Design review of the part built by this model. Coordinates are the model's own, in mm. A direction names the side the tool comes from. Give positions to 0.01 mm unless a question says otherwise; leave off trailing zeros. Order: outer loops, then holes, each group sorted by start corner. A loop starts at its lowest first (then second) coordinate and runs counter-clockwise, first axis right, second up. Notation, with made-up numbers: M -29.75,11 L -9.75,11 A18 ccw -9.75,36 Z; hole C -37,74 d1. An arc over 180 degrees is marked long. Answer as a JSON object with one key per item and string values.
from build123d import *

# Parameters (mm, degrees)
SKETCH_2_W          = 50
SKETCH_2_H          = 60
EXTRUDE_1_DEPTH     = 5
SKETCH_3_W          = 5
SKETCH_3_H          = 60
EXTRUDE_2_DEPTH     = 80
EXTRUDE_3_DEPTH     = 10
EXTRUDE_4_DEPTH     = 10
EXTRUDE_5_DEPTH     = 5
SKETCH_7_R          = 1.55
CUT_EXTRUDE_1_DEPTH = 112.803398875


with BuildPart() as part:
    # 草图2 → 凸台-拉伸1 (new body)
    with BuildSketch(Plane(origin=(0, 0, 0), x_dir=(1, 0, 0), z_dir=(0, 1, 0))):
        with Locations((25, 30)):
            Rectangle(SKETCH_2_W, SKETCH_2_H)
    extrude(amount=EXTRUDE_1_DEPTH)

    # 草图3 → 凸台-拉伸2 (add)
    with BuildSketch(Plane(origin=(0, 5, 0), x_dir=(1, 0, 0), z_dir=(0, 1, 0))):
        with Locations((47.5, 30)):
            Rectangle(SKETCH_3_W, SKETCH_3_H)
    extrude(amount=EXTRUDE_2_DEPTH)

    # 草图4 → 凸台-拉伸3 (add)
    with BuildSketch(Plane.XY):
        Polygon((39, 5), (45, 25), (45, 5), align=None)
    extrude(amount=-EXTRUDE_3_DEPTH)

    # 草图5 → 凸台-拉伸4 (add)
    with BuildSketch(Plane(origin=(0, 0, -60), x_dir=(-1, 0, 0), z_dir=(0, 0, -1))):
        Polygon((-39, 5), (-45, 25), (-45, 5), align=None)
    extrude(amount=-EXTRUDE_4_DEPTH)

    # 草图6 → 凸台-拉伸5 (add, symmetric)
    with BuildSketch(Plane(origin=(0, 0, -30), x_dir=(-1, 0, 0), z_dir=(0, 0, -1))):
        Polygon((-39, 5), (-45, 25), (-45, 5), align=None)
    extrude(amount=EXTRUDE_5_DEPTH, both=True)

    # 草图7 → 切除-拉伸1 (cut, through all)
    with BuildSketch(Plane(origin=(0, 5, 0), x_dir=(1, 0, 0), z_dir=(0, 1, 0))):
        with Locations(Location((6.5, 43, 0), (0, 0, 270))):
            Circle(SKETCH_7_R)
        with Locations(Location((32.5, 43, 0), (0, 0, 90))):
            Circle(SKETCH_7_R)
        with Locations(Location((6.5, 17, 0), (0, 0, 90))):
            Circle(SKETCH_7_R)
        with Locations(Location((32.5, 17, 0), (0, 0, 270))):
            Circle(SKETCH_7_R)
    extrude(amount=-CUT_EXTRUDE_1_DEPTH, mode=Mode.SUBTRACT)


solid = part.part
(1) We need section C-C (z = -29.5). Write out the cut boundary in (x, y), plus the area to 3 significant figures.
Checked values:
{"outline": "M 0,0 L 50,0 L 50,85 L 45,85 L 45,25 L 39,5 L 0,5 Z", "area": "710 mm^2"}
(2) Insertion check: pin 1 (10 mm diameter, centred on x = 24, z = -25.5, fed in from +Y); pin 2 (4 mm diameter, centred on y = 45.5, z = -28.5, fed in from -X). Each pin has a flat end and moves straight along its axis. Give the tip position at first contact, or say it passes through.
Checked values:
{"pin 1": "stops at y = 5", "pin 2": "stops at x = 45"}
(3) Tool access review of faces 5 (the flat face through (47, 85, -30)), 6 (the flat face through (43, 11, -50)): name each direction out of +Z, -Z, +X, -X, +Y, -Y from which nothing blocks a thin tool from reaching the whole face with its end or side.
Checked values:
{"face 5": "+Z, -Z, +X, -X, +Y", "face 6": "-X, +Y"}
(4) We need section B-B (x = 32.5). Write out the cut boundary in (y, z).
Checked values:
{"outline": "M 0,-60 L 5,-60 L 5,-44.55 L 0,-44.55 Z; M 0,-41.45 L 5,-41.45 L 5,-18.55 L 0,-18.55 Z; M 0,-15.45 L 5,-15.45 L 5,0 L 0,0 Z"}
(5) Draft analysis for pull direction X (two halves, no side actions). For faces 1 (the cylindrical face through (7.44, 2.54, -15.77)), 2 (the flat face through (43, 11, -35)), 3 (the flat face through (45, 44, -30)), 4 (the cylindrical face through (34.037, 2.535, -17.202)), state which applies: +X half, -X half, draft (parallel to the pull), parting line (faces both ways), or undercut.
Checked values:
{"face 1": "undercut", "face 2": "draft", "face 3": "-X half", "face 4": "undercut"}
(6) To check wall thickness, follow L1, parallel to X at y = 2, z = -43; L2, parallel to Y at x = 33, z = -36; L3, parallel to X at y = 46, z = -34. State the ranges of each line that lie inside material, in increasing order. Write a range as from..to.
Checked values:
{"L1": "x = 0..4.95, 8.05..30.95, 34.05..50", "L2": "y = 0..5", "L3": "x = 45..50"}
(7) We need section D-D (y = 17.5). Write out the cut boundary in (x, z).
Checked values:
{"outline": "M 42.75,-60 L 50,-60 L 50,0 L 42.75,0 L 42.75,-10 L 45,-10 L 45,-25 L 42.75,-25 L 42.75,-35 L 45,-35 L 45,-50 L 42.75,-50 Z"}
(8) We need section A-A (z = -17). Write out the cut boundary in (x, y), plus the area to 3 significant figures.
Checked values:
{"outline": "M 0,0 L 4.95,0 L 4.95,5 L 0,5 Z; M 8.05,0 L 30.95,0 L 30.95,5 L 8.05,5 Z; M 34.05,0 L 50,0 L 50,85 L 45,85 L 45,5 L 34.05,5 Z", "area": "619 mm^2"}
